```python
from build123d import *

# Parameters (mm, degrees)
SKETCH1_W           = 49
SKETCH1_H           = 30
BOSS_EXTRUDE1_DEPTH = 1
CUT_EXTRUDE1_DEPTH  = 10


with BuildPart() as part:
    # Sketch1 → Boss-Extrude1 (new body, symmetric)
    with BuildSketch(Plane.XY):
        Rectangle(SKETCH1_W, SKETCH1_H)
    extrude(amount=BOSS_EXTRUDE1_DEPTH, both=True)

    # Sketch2 → Cut-Extrude1 (cut)
    with BuildSketch(Plane.XY.offset(1)):
        with BuildLine():
            Line((-9.734337139, -14.270273119), (-17.013674651, -8.162183698))
            Line((-17.013674651, -8.162183698), (-16.692280846, -7.779161476))
            Line((-16.692280846, -7.779161476), (-9.412943334, -13.887250898))
            ThreePointArc((-9.412943334, -13.887250898), (-8.034845121, -12.536444461), (-6.465256226, -11.413847733))
            Line((-6.465256226, -11.413847733), (-16.471025722, 5.916653404))
            ThreePointArc((-16.471025722, 5.916653404), (-16.255, 6.042485877), (-16.038013021, 6.166653404))
            Line((-16.038013021, 6.166653404), (-6.032243524, -11.163847733))
            ThreePointArc((-6.032243524, -11.163847733), (-4.275251792, -10.36584224), (-2.416369995, -9.847777397))
            Line((-2.416369995, -9.847777397), (-5.891337274, 9.859741353))
            ThreePointArc((-5.891337274, 9.859741353), (-5.645302256, 9.90410005), (-5.398933397, 9.946565442))
            Line((-5.398933397, 9.946565442), (-1.923966119, -9.760953309))
            ThreePointArc((-1.923966119, -9.760953309), (0, -9.612), (1.923966119, -9.760953309))
            Line((1.923966119, -9.760953309), (5.398933397, 9.946565442))
            ThreePointArc((5.398933397, 9.946565442), (5.645302256, 9.90410005), (5.891337274, 9.859741353))
            Line((5.891337274, 9.859741353), (2.416369995, -9.847777397))
            ThreePointArc((2.416369995, -9.847777397), (4.275251792, -10.36584224), (6.032243524, -11.163847733))
            Line((6.032243524, -11.163847733), (16.038013021, 6.166653404))
            ThreePointArc((16.038013021, 6.166653404), (16.255, 6.042485877), (16.471025722, 5.916653404))
            Line((16.471025722, 5.916653404), (6.465256226, -11.413847733))
            ThreePointArc((6.465256226, -11.413847733), (8.034845121, -12.536444461), (9.412943334, -13.887250898))
            Line((9.412943334, -13.887250898), (16.692280846, -7.779161476))
            Line((16.692280846, -7.779161476), (17.013674651, -8.162183698))
            Line((17.013674651, -8.162183698), (9.734337139, -14.270273119))
            ThreePointArc((9.734337139, -14.270273119), (10.013600489, -14.630168322), (10.279564971, -15))
            Line((10.279564971, -15), (-10.279564971, -15))
            ThreePointArc((-10.279564971, -15), (-10.013600489, -14.630168322), (-9.734337139, -14.270273119))
        make_face()
    extrude(amount=-CUT_EXTRUDE1_DEPTH, mode=Mode.SUBTRACT)


solid = part.part
```
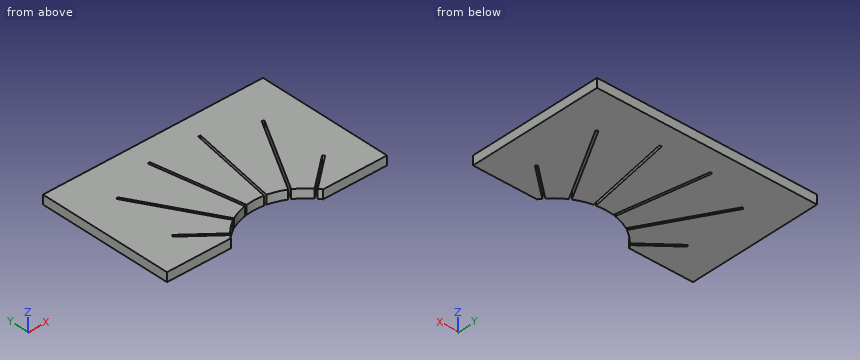
Source: CAD feature listing. Evaluate the final solid. Frame: model axes, mm. Round coordinates to 2 decimals unless told otherwise and drop trailing zeros. Loops run counter-clockwise (first coordinate to the right, second up) from the corner with the lowest first, then second, coordinate; pieces in that order, holes last.
(1) Section query B-B (x = 7.5). Output: boundary loops of the cut face in (y, z).
From the geometry:
outline: (-12.11, -1) - (-9.62, -1) - (-9.62, 1) - (-12.11, 1) - close; (-8.62, -1) - (15, -1) - (15, 1) - (-8.62, 1) - close
(2) Section query D-D (y = 1). Output: boundary loops of the cut face in (x, z).
From the geometry:
outline: (-24.5, -1) - (-13.63, -1) - (-13.63, 1) - (-24.5, 1) - close; (-13.06, -1) - (-4.33, -1) - (-4.33, 1) - (-13.06, 1) - close; (-3.82, -1) - (3.82, -1) - (3.82, 1) - (-3.82, 1) - close; (4.33, -1) - (13.06, -1) - (13.06, 1) - (4.33, 1) - close; (13.63, -1) - (24.5, -1) - (24.5, 1) - (13.63, 1) - close
(3) Material intervals for probe 1 along Y at (x, z) = (16, 0.8); probe 2 along X at (y, z) = (7.25, 0); probe 3 along Y at (x, z) = (-15.5, 0.25), sorted ascending.
From the geometry:
probe 1: y = -15 to -9.01, -8.36 to 5.1, 6.1 to 15
probe 2: x = -24.5 to -5.43, -4.92 to 4.92, 5.43 to 24.5
probe 3: y = -15 to -9.43, -8.78 to 4.23, 5.23 to 15
(4) Section query A-A (y = 7). Output: boundary loops of the cut face in (x, z).
From the geometry:
outline: (-24.5, -1) - (-5.39, -1) - (-5.39, 1) - (-24.5, 1) - close; (-4.88, -1) - (4.88, -1) - (4.88, 1) - (-4.88, 1) - close; (5.39, -1) - (24.5, -1) - (24.5, 1) - (5.39, 1) - close
